The drawing under review shows one solid part. Ordinate dimensions are in mm from its lowest x, y, z. Coordinates: 2 decimals unless noted, no trailing zeros. Write each loop counter-clockwise with the first axis right and the second up, starting at its lowest first coordinate (ties: lowest second). Pieces come first, ordered by that corner, then holes. Notation, with made-up numbers: (35, -6) -> (75, -6) arc R15 cw to (75, 15) -> close; hole circle Ø3 at (78.25, 6). An arc over 180 degrees is marked (long way). One line per question, with ' | ' between items. Start each with the question number.
Q1. For P1, Ø5, axis at x = 38.14, y = 14.75, coming from the -Z side; P2, Ø3.5, axis at x = 52.86, y = 14.75, coming from the +Z side, all flat-tipped, find the tip position at first contact; note any pin that passes through.
Q2. Add section D-D on x = 55.5. State the section outline as (y, z) points, and give its area (3 significant figures).
Q3. Wall thickness on probe 1 along X at (y, z) = (14.75, 1.15); probe 2 along X at (y, z) = (27.5, 1); probe 3 along Y at (x, z) = (43, 4.5): over which ranges is each line inside the solid? List them lowest first.
Q4. Add section B-B on y = 19. State the section outline as (x, z) points, and give its area (3 significant figures).
Q5. Add section C-C on z = 4.5. State the section outline as (x, y) points.
Q6. Add section A-A on x = 45.5. State the section outline as (y, z) points.
Q7. Draft analysis for pull direction Y (two halves, no side actions). For the marked faces 1, 2 and 3, state which applies: pulls with the +Y half, pulls with the -Y half, needs draft (parallel to the pull), parting line crosses it, or undercut.
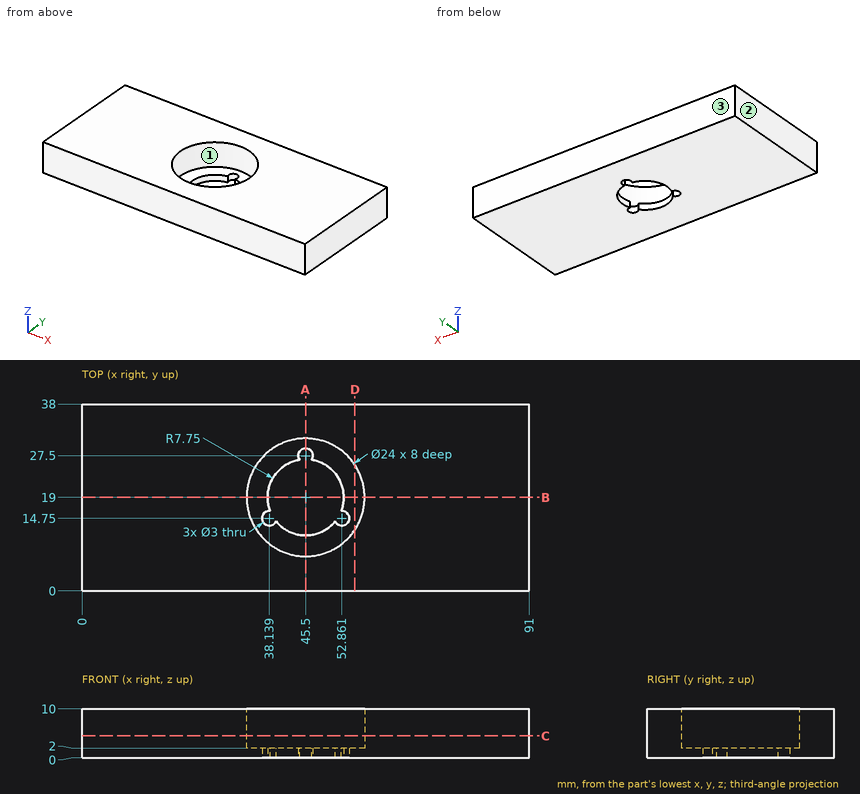
Output values:
1) P1: stops at z = 0 | P2: stops at z = 2
2) outline: (0, 0) -> (38, 0) -> (38, 10) -> (25.63, 10) -> (25.63, 2) -> (12.37, 2) -> (12.37, 10) -> (0, 10) -> close | area: 274 mm2
3) probe 1: x = 0 to 36.64, 54.36 to 91 | probe 2: x = 0 to 44, 47 to 91 | probe 3: y = 0 to 7.26, 30.74 to 38
4) outline: (0, 0) -> (37.75, 0) -> (37.75, 2) -> (33.5, 2) -> (33.5, 10) -> (0, 10) -> close; (53.25, 0) -> (91, 0) -> (91, 10) -> (57.5, 10) -> (57.5, 2) -> (53.25, 2) -> close | area: 687 mm2
5) outline: (0, 0) -> (91, 0) -> (91, 38) -> (0, 38) -> close; hole circle Ø24 at (45.5, 19)
6) outline: (0, 0) -> (11.25, 0) -> (11.25, 2) -> (7, 2) -> (7, 10) -> (0, 10) -> close; (29, 0) -> (38, 0) -> (38, 10) -> (31, 10) -> (31, 2) -> (29, 2) -> close
7) face 1: undercut | face 2: needs draft | face 3: pulls with the +Y half
